Design review of the part built by this model. Coordinates are the model's own, in mm. Face numbers are marked on the shaded views. A direction names the side the tool comes from. Round coordinates to 2 decimals unless told otherwise and drop trailing zeros. Loops run counter-clockwise (first coordinate to the right, second up) from the corner with the lowest first, then second, coordinate; pieces in that order, holes last. Notation, with made-up numbers: (74, 25) - (81, 25) arc R26 cw to (81, 62) - close; hole circle Ø6 at (58, 15). An arc over 180 degrees is marked (long way). Answer as CSV lines item,"result". Start each with the question number.
(1) Wall thickness on L1, parallel to Y at x = -23, z = 5; L2, parallel to X at y = 3, z = 7.75; L3, parallel to Y at x = -8.5, z = 8: over which ranges is each line inside the solid? List them lowest first.
(2) Mouldability with a two-part tool opening along Y and no side actions: class the marked faces 1, 2, 3 and 4 as released by +Y, released by -Y, zero draft, split by the parting line, or undercut.
(3) Consider section B-B (z = 2.5). Give the boundary of the cut face in (x, y), and give its area (3 significant figures).
(4) Consider section A-A (y = 0). Give the boundary of the cut face in (x, z) (3 decimals).
(5) Consider section C-C (x = -8). Give the boundary of the cut face in (y, z), and give its area (3 significant figures).
(6) For P1, Ø4, axis at x = -7, y = 2.5, coming from the -Z side; P2, Ø1.5, axis at x = 17.5, y = 0.5, coming from the -Z side; P3, Ø12, axis at x = -3, y = 1, coming from the +Z side; P4, Ø5.5, axis at x = 24, y = -7.5, coming from the +Z side, all flat-tipped, find the tip position at first contact; note any pin that passes through.
(7) For the marked faces 5, 6 and 7, list the 3-axis set-ups (+Z, -Z, +X, -X, +Y, -Y) from which the entire face can be reached by the end or side of a thin tool; tool diameter is ignored.
(8) Consider section D-D (x = 0). Give the boundary of the cut face in (y, z).
from build123d import *

# Parameters (mm, degrees)
F0_W     = 42
F0_H     = 19.5
F0_R     = 7.5
F1_DEPTH = 1
F2_W     = 42
F2_H     = 5
F3_DEPTH = 10
F4_DEPTH = 9


with BuildPart() as f1:
    # F0 (on Top) → F1 (new body)
    with BuildSketch(Plane.XY):
        Rectangle(F0_W, F0_H)
        Polygon((0.75, 8.25), (0.75, 0), (0.75, -8.25), (-18.5, -8.25), (-18.5, 8.25), align=None, mode=Mode.SUBTRACT)
        Polygon((0.75, -8.25), (0.75, 0), (0.75, 8.25), (-18.5, 8.25), (-18.5, -8.25), align=None)
        with Locations((-10.125, 0)):
            Circle(F0_R, mode=Mode.SUBTRACT)
    extrude(amount=F1_DEPTH)

    # F2 (on Top) → F3 (join)
    with BuildSketch(Plane.XY):
        with Locations((0, 12.25)):
            Rectangle(F2_W, F2_H)
        with Locations((0, -12.25)):
            Rectangle(F2_W, F2_H)
    extrude(amount=F3_DEPTH)

    # F2 (on Top) → F4 (join)
    with BuildSketch(Plane.XY):
        Polygon((-21, -9.75), (-21, -0.75), (-26, -0.75), (-26, -14.75), (-21, -14.75), align=None)
        Polygon((26, 14.75), (21, 14.75), (21, 9.75), (21, 0.75), (26, 0.75), align=None)
        Polygon((26, -0.75), (21, -0.75), (21, -9.75), (21, -14.75), (26, -14.75), align=None)
        Polygon((-21, 9.75), (-21, 14.75), (-26, 14.75), (-26, 0.75), (-21, 0.75), align=None)
    extrude(amount=F4_DEPTH)


solid = f1.part
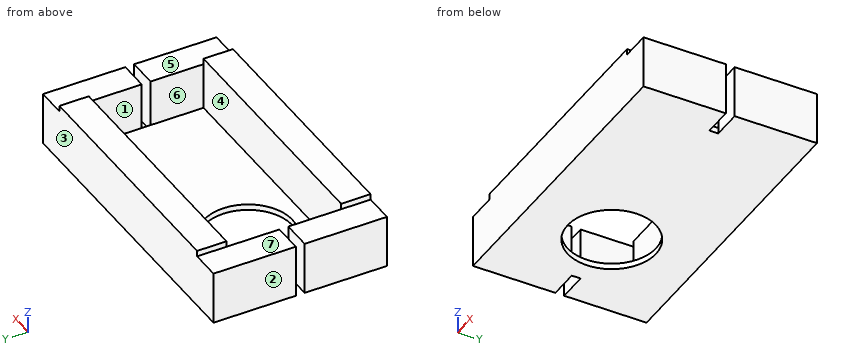
Determined:
1,L1,"y = -14.75 to -0.75, 0.75 to 14.75"
1,L2,"x = -26 to -21, 21 to 26"
1,L3,"y = -14.75 to -9.75, 9.75 to 14.75"
2,face 1,"undercut"
2,face 2,"zero draft"
2,face 3,"released by +Y"
2,face 4,"undercut"
3,outline,"(-26, -14.75) - (26, -14.75) - (26, -0.75) - (21, -0.75) - (21, -9.75) - (-21, -9.75) - (-21, -0.75) - (-26, -0.75) - close; (-26, 0.75) - (-21, 0.75) - (-21, 9.75) - (21, 9.75) - (21, 0.75) - (26, 0.75) - (26, 14.75) - (-26, 14.75) - close"
3,area,"700 mm^2"
4,outline,"(-21, 0) - (-17.625, 0) - (-17.625, 1) - (-21, 1) - close; (-2.625, 0) - (21, 0) - (21, 1) - (-2.625, 1) - close"
5,outline,"(-14.75, 0) - (-7.19, 0) - (-7.19, 1) - (-9.75, 1) - (-9.75, 10) - (-14.75, 10) - close; (7.19, 0) - (14.75, 0) - (14.75, 10) - (9.75, 10) - (9.75, 1) - (7.19, 1) - close"
5,area,"105 mm^2"
6,P1,"passes through"
6,P2,"stops at z = 0"
6,P3,"stops at z = 1"
6,P4,"stops at z = 9"
7,face 5,"+Z, +X, +Y, -Y"
7,face 6,"+Z"
7,face 7,"+Z, -X, +Y, -Y"
8,outline,"(-14.75, 0) - (14.75, 0) - (14.75, 10) - (9.75, 10) - (9.75, 1) - (-9.75, 1) - (-9.75, 10) - (-14.75, 10) - close"
